from build123d import *

# Parameters (mm, degrees)
SKETCH1_W                   = 250
SKETCH1_H                   = 170
BOSS_EXTRUDE3_DEPTH         = 65
CUT_EXTRUDE1_START          = 4
SKETCH1_3_W                 = 150
SKETCH1_3_H                 = 65
CUT_EXTRUDE1_DEPTH          = 166.92645468
SKETCH6_W                   = 230
SKETCH6_H                   = 150
SKETCH6_W_2                 = 170
SKETCH6_H_2                 = 85
CUT_EXTRUDE2_DEPTH          = 55
SKETCH7_W                   = 144
SKETCH7_H                   = 59
CUT_EXTRUDE3_DEPTH          = 169.436931817
TAP_DRILL_FOR_M3_TAP1_D     = 2.5
TAP_DRILL_FOR_M3_TAP1_DEPTH = 5
TAP_DRILL_FOR_M3_TAP1_TIP   = 0.751075774
TAP_DRILL_FOR_M3_TAP3_D     = 2.5
TAP_DRILL_FOR_M3_TAP3_DEPTH = 5
TAP_DRILL_FOR_M3_TAP3_TIP   = 0.751075774
FILLET3_R                   = 10
CUT_EXTRUDE4_START          = -10
SKETCH19_W                  = 250
SKETCH19_H                  = 170
CUT_EXTRUDE4_DEPTH          = 10
FILLET2_R                   = 2
CHAMFER1_SIZE               = 1
CHAMFER2_SIZE               = 10


with BuildPart() as part:
    # Sketch1 → Boss-Extrude3 (new body)
    with BuildSketch(Plane.XY):
        with Locations((0, 10)):
            Rectangle(SKETCH1_W, SKETCH1_H)
    extrude(amount=BOSS_EXTRUDE3_DEPTH)

    # Sketch1<3> → Cut-Extrude1 (cut, through all)
    with BuildSketch(Plane.XY.offset(CUT_EXTRUDE1_START)):
        Rectangle(SKETCH1_3_W, SKETCH1_3_H)
    extrude(amount=CUT_EXTRUDE1_DEPTH, mode=Mode.SUBTRACT)

    # Sketch6 → Cut-Extrude2 (cut)
    with BuildSketch(Plane.XY.offset(65)):
        with Locations((0, 10)):
            Rectangle(SKETCH6_W, SKETCH6_H)
        Rectangle(SKETCH6_W_2, SKETCH6_H_2, mode=Mode.SUBTRACT)
    extrude(amount=-CUT_EXTRUDE2_DEPTH, mode=Mode.SUBTRACT)

    # Sketch7 → Cut-Extrude3 (cut, through all)
    with BuildSketch(Plane.XY.offset(4)):
        Rectangle(SKETCH7_W, SKETCH7_H)
    extrude(amount=-CUT_EXTRUDE3_DEPTH, mode=Mode.SUBTRACT)

    # Tap Drill for M3 Tap1
    with Locations(Plane(origin=(0, -75, 0), x_dir=(-1, 0, 0), z_dir=(0, -1, 0))):
        with Locations((-60, -5), (0, -5), (60, -5)):
            Hole(TAP_DRILL_FOR_M3_TAP1_D / 2, depth=TAP_DRILL_FOR_M3_TAP1_DEPTH)
            with Locations((0, 0, -(TAP_DRILL_FOR_M3_TAP1_DEPTH + TAP_DRILL_FOR_M3_TAP1_TIP / 2))):  # 118° drill point
                Cone(0, TAP_DRILL_FOR_M3_TAP1_D / 2, TAP_DRILL_FOR_M3_TAP1_TIP, mode=Mode.SUBTRACT)

    # Tap Drill for M3 Tap3
    with Locations(Plane.ZY.offset(125)):
        with Locations((5, 60), (5, 0), (5, -60)):
            Hole(TAP_DRILL_FOR_M3_TAP3_D / 2, depth=TAP_DRILL_FOR_M3_TAP3_DEPTH)
            with Locations((0, 0, -(TAP_DRILL_FOR_M3_TAP3_DEPTH + TAP_DRILL_FOR_M3_TAP3_TIP / 2))):  # 118° drill point
                Cone(0, TAP_DRILL_FOR_M3_TAP3_D / 2, TAP_DRILL_FOR_M3_TAP3_TIP, mode=Mode.SUBTRACT)

    # Fillet3
    fillet3_edges = [part.edges().sort_by_distance(p)[0] for p in [
        (115, -65, 37.5),
        (115, 85, 37.5),
        (-115, 85, 37.5),
        (-115, -65, 37.5),
        (-72, -29.5, 2),
        (-72, 29.5, 2),
        (72, 29.5, 2),
        (72, -29.5, 2),
    ]]
    fillet(fillet3_edges, radius=FILLET3_R)

    # Sketch19 → Cut-Extrude4 (cut)
    with BuildSketch(Plane.XY.offset(65).offset(CUT_EXTRUDE4_START)):
        with Locations((0, 10)):
            Rectangle(SKETCH19_W, SKETCH19_H)
        with BuildLine():
            Line((-115, 75), (-115, -55))
            ThreePointArc((-115, -55), (-112.071067812, -62.071067812), (-105, -65))
            Line((-105, -65), (105, -65))
            ThreePointArc((105, -65), (112.071067812, -62.071067812), (115, -55))
            Line((115, -55), (115, 75))
            ThreePointArc((115, 75), (112.071067812, 82.071067812), (105, 85))
            Line((105, 85), (-105, 85))
            ThreePointArc((-105, 85), (-112.071067812, 82.071067812), (-115, 75))
        make_face(mode=Mode.SUBTRACT)
    extrude(amount=CUT_EXTRUDE4_DEPTH, mode=Mode.SUBTRACT)

    # Fillet2
    fillet2_edges = [part.edges().sort_by_distance(p)[0] for p in [
        (-75, 32.5, 34.5),
        (-75, -32.5, 34.5),
        (75, -32.5, 34.5),
        (75, 32.5, 34.5),
    ]]
    fillet(fillet2_edges, radius=FILLET2_R)

    # Chamfer1
    chamfer1_edges = [part.edges().sort_by_distance(p)[0] for p in [
        (-75, 0, 65),
        (0, -32.5, 65),
        (75, 0, 65),
        (0, 32.5, 65),
        (-74.414213562, -31.914213562, 65),
        (74.414213562, -31.914213562, 65),
        (74.414213562, 31.914213562, 65),
        (-74.414213562, 31.914213562, 65),
    ]]
    chamfer(chamfer1_edges, length=CHAMFER1_SIZE)

    # Chamfer2
    chamfer2_edges = [part.edges().sort_by_distance(p)[0] for p in [
        (125, 95, 27.5),
    ]]
    chamfer(chamfer2_edges, length=CHAMFER2_SIZE)


solid = part.part
For this review, take the finished solid that the model builds, in its own axes (mm). A direction names the side the tool comes from. Round coordinates to 2 decimals unless told otherwise and drop trailing zeros. Order: outer loops, then holes, each group sorted by start corner. A loop starts at its lowest first (then second) coordinate and runs counter-clockwise, first axis right, second up. Notation, with made-up numbers: M -36.75,68 L 12.25,68 A27 ccw 12.25,97 Z; hole C 21,31.5 d11. An arc over 180 degrees is marked long. Use a Markdown table: item, result. Add a question column.
Item 1: To check wall thickness, follow line 1 along X through (y, z) = (-71, 5); line 2 along Y through (x, z) = (-48, 50); line 3 along Y through (x, z) = (-123, 5). State the ranges of each line that lie inside material, in increasing order.
Item 2: Insertion check: pin 1 (6 mm diameter, centred on x = -90.5, y = 53, fed in from +Z); pin 2 (4 mm diameter, centred on y = -28.5, z = 57.5, fed in from +X). Each pin has a flat end and moves straight along its axis. Give the tip position at first contact, or say it passes through.
Item 3: Add section A-A, the plane z = 35. Give the boundary of the cut face in (x, y), then the cut area to 3 significant figures.
Item 4: Add section B-B, the plane x = 101.5. Give the boundary of the cut face in (y, z).
Item 5: Tool access review of faces 1 (the flat face through (-85, -1, 38)), 2 (the cylindrical face through (-68.99, 26.65, 1.97)), 3 (the flat face through (120, 90, 27)): name each direction out of +Z, -Z, +X, -X, +Y, -Y from which nothing blocks a thin tool from reaching the whole face with its end or side.
Item 6: Add section C-C, the plane z = 60. Give the boundary of the cut face in (x, y), then the cut area to 3 significant figures.
Geometry results:
| question | item | result |
|---|---|---|
| 1 | line 1 | x = -125 to -61.25, -58.75 to -1.25, 1.25 to 58.75, 61.25 to 125 |
| 1 | line 2 | y = -75 to -65, -42.5 to -32.5, 32.5 to 42.5, 85 to 95 |
| 1 | line 3 | y = -75 to -61.25, -58.75 to -1.25, 1.25 to 58.75, 61.25 to 95 |
| 2 | pin 1 | stops at z = 10 |
| 2 | pin 2 | stops at x = 85 |
| 3 | outline | M -125,-75 L 125,-75 L 125,85 L 115,95 L -125,95 Z; M -85,-42.5 L 85,-42.5 L 85,42.5 L -85,42.5 Z; hole M -115,-55 A10 ccw -105,-65 L 105,-65 A10 ccw 115,-55 L 115,75 A10 ccw 105,85 L -105,85 A10 ccw -115,75 Z; hole M -75,-30.5 A2 ccw -73,-32.5 L 73,-32.5 A2 ccw 75,-30.5 L 75,30.5 A2 ccw 73,32.5 L -73,32.5 A2 ccw -75,30.5 Z |
| 3 | area | 12,700 mm² |
| 4 | outline | M -75,0 L 95,0 L 95,55 L 85,55 L 85,10 L -65,10 L -65,55 L -75,55 Z |
| 5 | face 1 | +Z |
| 5 | face 2 | +Z, -Z |
| 5 | face 3 | +Z, -Z, +X, +Y |
| 6 | outline | M -85,-42.5 L 85,-42.5 L 85,42.5 L -85,42.5 Z; hole M -75,-30.5 A2 ccw -73,-32.5 L 73,-32.5 A2 ccw 75,-30.5 L 75,30.5 A2 ccw 73,32.5 L -73,32.5 A2 ccw -75,30.5 Z |
| 6 | area | 4,700 mm² |
